from build123d import *

# Parameters (mm, degrees)
CROQUIS1_W                 = 37.5
CROQUIS1_H                 = 30
SALIENTE_EXTRUIR1_DEPTH    = 15
CROQUIS2_R                 = 2.1
SALIENTE_EXTRUIR2_DEPTH    = 1
SALIENTE_EXTRUIR3_DEPTH    = 35
CROQUIS5_W                 = 18
CROQUIS5_H                 = 12
CROQUIS5_R                 = 4.5
SALIENTE_EXTRUIR4_DEPTH    = 5
CROQUIS6_W                 = 1
CROQUIS6_H                 = 12
CORTAR_EXTRUIR2_DEPTH      = 14
REDONDEO1_R                = 3
REDONDEO2_R                = 3
CORTAR_EXTRUIR3_DEPTH      = 78.447159406
CORTAR_EXTRUIR3_DEPTH_BACK = 78.447159406
CROQUIS7_OUTSIDE_W         = 123.972
CROQUIS7_OUTSIDE_H         = 74.472
CROQUIS7_OUTSIDE_W_2       = 24.163279834
CROQUIS7_OUTSIDE_H_2       = 36.211204922
SALIENTE_EXTRUIR5_DEPTH    = 147.5


with BuildPart() as part:
    # Croquis1 → Saliente-Extruir1 (new body)
    with BuildSketch(Plane.XY):
        Rectangle(CROQUIS1_W, CROQUIS1_H)
    extrude(amount=SALIENTE_EXTRUIR1_DEPTH)

    # Croquis2 → Saliente-Extruir2 (add)
    # profile 1 of 3: a face of its own
    with BuildSketch(Plane.XY):
        with BuildLine():
            Line((-18.75, 3.7), (-26.75, 3.7))
            ThreePointArc((-26.75, 3.7), (-27.457106781, 3.407106781), (-27.75, 2.7))
            Line((-27.75, 2.7), (-27.75, -2.7))
            ThreePointArc((-27.75, -2.7), (-27.457106781, -3.407106781), (-26.75, -3.7))
            Line((-26.75, -3.7), (-18.75, -3.7))
            Line((-18.75, -3.7), (-18.75, 3.7))
        make_face()
        with Locations((-23.25, 0)):
            Circle(CROQUIS2_R, mode=Mode.SUBTRACT)
    # profile 2 of 3: a face of its own
    with BuildSketch(Plane.XY):
        with BuildLine():
            Line((-10, 15), (10, 15))
            Line((10, 15), (10, 24))
            ThreePointArc((10, 24), (9.707106781, 24.707106781), (9, 25))
            Line((9, 25), (-9, 25))
            ThreePointArc((-9, 25), (-9.707106781, 24.707106781), (-10, 24))
            Line((-10, 24), (-10, 15))
        make_face()
        with Locations((-5.5, 20)):
            Circle(CROQUIS2_R, mode=Mode.SUBTRACT)
        with Locations((5.5, 20)):
            Circle(CROQUIS2_R, mode=Mode.SUBTRACT)
    # profile 3 of 3: a face of its own
    with BuildSketch(Plane.XY):
        with BuildLine():
            Line((-9, -25), (9, -25))
            ThreePointArc((9, -25), (9.707106781, -24.707106781), (10, -24))
            Line((10, -24), (10, -15))
            Line((10, -15), (-10, -15))
            Line((-10, -15), (-10, -24))
            ThreePointArc((-10, -24), (-9.707106781, -24.707106781), (-9, -25))
        make_face()
        with Locations(Location((5.5, -20, 0), (0, 0, 180))):
            Circle(CROQUIS2_R, mode=Mode.SUBTRACT)
        with Locations(Location((-5.5, -20, 0), (0, 0, 180))):
            Circle(CROQUIS2_R, mode=Mode.SUBTRACT)
    extrude(amount=SALIENTE_EXTRUIR2_DEPTH)

    # Croquis3 → Saliente-Extruir3 (add)
    with BuildSketch(Plane(origin=(18.75, 0, 0), x_dir=(0, 0, -1), z_dir=(1, 0, 0))):
        with BuildLine():
            Line((-10.5, -12.5), (-4.5, -12.5))
            ThreePointArc((-4.5, -12.5), (-2.378679656, -11.621320344), (-1.5, -9.5))
            Line((-1.5, -9.5), (-1.5, 9.5))
            ThreePointArc((-1.5, 9.5), (-2.378679656, 11.621320344), (-4.5, 12.5))
            Line((-4.5, 12.5), (-10.5, 12.5))
            ThreePointArc((-10.5, 12.5), (-12.621320344, 11.621320344), (-13.5, 9.5))
            Line((-13.5, 9.5), (-13.5, -9.5))
            ThreePointArc((-13.5, -9.5), (-12.621320344, -11.621320344), (-10.5, -12.5))
        make_face()
    extrude(amount=SALIENTE_EXTRUIR3_DEPTH)

    # Croquis5 → Saliente-Extruir4 (add, symmetric)
    with BuildSketch(Plane.XY.offset(7.5)):
        with Locations((62.75, 0)):
            Rectangle(CROQUIS5_W, CROQUIS5_H)
        with Locations((64.25, 0)):
            Circle(CROQUIS5_R, mode=Mode.SUBTRACT)
    extrude(amount=SALIENTE_EXTRUIR4_DEPTH, both=True)

    # Croquis6 → Cortar-Extruir2 (cut)
    with BuildSketch(Plane(origin=(71.75, 0, 0), x_dir=(0, 0, -1), z_dir=(1, 0, 0))):
        with Locations((-12, 0)):
            Rectangle(CROQUIS6_W, CROQUIS6_H)
        with Locations((-3, 0)):
            Rectangle(CROQUIS6_W, CROQUIS6_H)
    extrude(amount=-CORTAR_EXTRUIR2_DEPTH, mode=Mode.SUBTRACT)

    # Redondeo1
    redondeo1_edges = [part.edges().sort_by_distance(p)[0] for p in [
        (71.75, 6, 7.5),
        (71.75, -6, 7.5),
    ]]
    fillet(redondeo1_edges, radius=REDONDEO1_R)

    # Redondeo2
    # the kernel refuses this fillet: 3 mm, written as the material it takes off along each edge
    with BuildSketch(Plane(origin=(75.75, -6, 12.5), x_dir=(0, 1, 0), z_dir=(-1, 0, 0)), Plane(origin=(53.75, 6, 2.5), x_dir=(0, 0, 1), z_dir=(1, 0, 0))) as redondeo2_piece_1:
        with BuildLine():
            CenterArc((REDONDEO2_R, REDONDEO2_R), REDONDEO2_R, 180, 90)
            Line((0, REDONDEO2_R), (-REDONDEO2_R * 0.02, REDONDEO2_R))
            Line((-REDONDEO2_R * 0.02, REDONDEO2_R), (-REDONDEO2_R * 0.02, -REDONDEO2_R * 0.02))
            Line((-REDONDEO2_R * 0.02, -REDONDEO2_R * 0.02), (REDONDEO2_R, -REDONDEO2_R * 0.02))
            Line((REDONDEO2_R, -REDONDEO2_R * 0.02), (REDONDEO2_R, 0))
        make_face()
    extrude(amount=22, mode=Mode.SUBTRACT)
    with BuildSketch(Plane(origin=(75.75, -6, 2.5), x_dir=(0, 1, 0), z_dir=(-1, 0, 0)), Plane(origin=(53.75, 6, 12.5), x_dir=(0, 0, -1), z_dir=(1, 0, 0))) as redondeo2_piece_2:
        with BuildLine():
            CenterArc((REDONDEO2_R, -REDONDEO2_R), REDONDEO2_R, 90, 90)
            Line((0, -REDONDEO2_R), (-REDONDEO2_R * 0.02, -REDONDEO2_R))
            Line((-REDONDEO2_R * 0.02, -REDONDEO2_R), (-REDONDEO2_R * 0.02, REDONDEO2_R * 0.02))
            Line((-REDONDEO2_R * 0.02, REDONDEO2_R * 0.02), (REDONDEO2_R, REDONDEO2_R * 0.02))
            Line((REDONDEO2_R, REDONDEO2_R * 0.02), (REDONDEO2_R, 0))
        make_face()
    extrude(amount=22, mode=Mode.SUBTRACT)

    # Croquis7 outside → Cortar-Extruir3 (cut, two sides: drawn at the far end of the back side and taken through both)
    with BuildSketch(Plane.XY.offset(15).offset(-CORTAR_EXTRUIR3_DEPTH_BACK)):
        with Locations((22, 0)):
            Rectangle(CROQUIS7_OUTSIDE_W, CROQUIS7_OUTSIDE_H)
        with Locations((65.831639917, -3.105602461)):
            Rectangle(CROQUIS7_OUTSIDE_W_2, CROQUIS7_OUTSIDE_H_2, mode=Mode.SUBTRACT)
    extrude(amount=CORTAR_EXTRUIR3_DEPTH + CORTAR_EXTRUIR3_DEPTH_BACK, mode=Mode.SUBTRACT)

    # Croquis10 → Saliente-Extruir5 (add)
    with BuildSketch(Plane.ZY.offset(-53.75)):
        with BuildLine():
            Line((5.5, -6), (9.5, -6))
            ThreePointArc((9.5, -6), (11.621320344, -5.121320344), (12.5, -3))
            Line((12.5, -3), (12.5, 3))
            ThreePointArc((12.5, 3), (11.621320344, 5.121320344), (9.5, 6))
            Line((9.5, 6), (5.5, 6))
            ThreePointArc((5.5, 6), (3.378679656, 5.121320344), (2.5, 3))
            Line((2.5, 3), (2.5, -3))
            ThreePointArc((2.5, -3), (3.378679656, -5.121320344), (5.5, -6))
        make_face()
    extrude(amount=SALIENTE_EXTRUIR5_DEPTH)


solid = part.part
The listing builds one solid part. Answer for the finished solid, in the listing's coordinates (mm). A direction names the side the tool comes from. Round coordinates to 2 decimals unless told otherwise and drop trailing zeros. Order: outer loops, then holes, each group sorted by start corner. A loop starts at its lowest first (then second) coordinate and runs counter-clockwise, first axis right, second up. Notation, with made-up numbers: (27.5, 64.25) - (60.5, 64.25) arc R22 cw to (60.5, 78.25) - close; hole circle Ø2 at (8, 1.25). An arc over 180 degrees is marked (long way). Write item = value, one per line. Start each with the question number.
1) Straight lines are drawn through the part: L1, parallel to Y at x = 64.25, z = 7.5; L2, parallel to X at y = 0, z = 6.5; L3, parallel to X at y = 1.5, z = 6.25. For each, find the intervals that lie inside material, in ascending order.
2) Section B-B, the plane x = 64.25 is taken. Write down the section's boundary in (y, z), plus the area to 3 significant figures.
3) For faces 1 (the flat face through (70, 0, 11.5)), 2 (the cylindrical face through (-10.35, 5.1, 11.64)), 3 (the flat face through (70, 0, 3.5)), determine the directions among +Z, -Z, +X, -X, +Y, -Y from which every point of the face is accessible in a straight line to the end or side of a thin tool.
4) Given pin 1 (4 mm diameter, centred on x = 15, z = 4, fed in from +Y); pin 2 (1.5 mm diameter, centred on x = -73.5, z = 4, fed in from -Y), each flat-ended and moving along its own axis, determine where each tip first touches the part or whether it passes through.
5) Section D-D, the plane x = -26 is taken. Write down the section's boundary in (y, z).
6) Section A-A, the plane z = 7.75 is taken. Write down the section's boundary in (x, y).
7) Section C-C, the plane y = 0 is taken. Write down the section's boundary in (x, z).
Results list:
q1.L1 = -6 to -4.5, 4.5 to 6
q1.L2 = -93.75 to 59.75, 68.75 to 71.75
q1.L3 = -93.75 to 60.01, 68.49 to 71.75
q2.outline = (-6, 5.5) arc R3 ccw to (-5.24, 3.5) - (-4.5, 3.5) - (-4.5, 11.5) - (-5.24, 11.5) arc R3 ccw to (-6, 9.5) - close; (4.5, 3.5) - (5.24, 3.5) arc R3 ccw to (6, 5.5) - (6, 9.5) arc R3 ccw to (5.24, 11.5) - (4.5, 11.5) - close
q2.area = 22.1 mm^2
q3.face_1 = +Z, +X, +Y, -Y
q3.face_2 = +Z, +X, -X, +Y
q3.face_3 = -Z, +X, +Y, -Y
q4.pin_1 = 6
q4.pin_2 = -5.9
q5.outline = (-6, 5.5) arc R3 ccw to (-3, 2.5) - (3, 2.5) arc R3 ccw to (6, 5.5) - (6, 9.5) arc R3 ccw to (3, 12.5) - (-3, 12.5) arc R3 ccw to (-6, 9.5) - close
q6.outline = (-93.75, -6) - (68.75, -6) arc R3 ccw to (71.75, -3) - (71.75, 3) arc R3 ccw to (68.75, 6) - (-93.75, 6) - close; hole circle Ø9 at (64.25, 0)
q7.outline = (-93.75, 2.5) - (57.75, 2.5) - (57.75, 3.5) - (59.75, 3.5) - (59.75, 11.5) - (57.75, 11.5) - (57.75, 12.5) - (-93.75, 12.5) - close; (68.75, 3.5) - (71.75, 3.5) - (71.75, 11.5) - (68.75, 11.5) - close
